For this review, take the finished solid that the model builds, in its own axes (mm). Round coordinates to 2 decimals unless told otherwise and drop trailing zeros. Write each loop counter-clockwise with the first axis right and the second up, starting at its lowest first coordinate (ties: lowest second). Pieces come first, ordered by that corner, then holes. Notation, with made-up numbers: M 50.25,-22.75 L 66.25,-22.75 A11 ccw 66.25,-14.75 Z; hole C -3.5,-0.75 d5. An arc over 180 degrees is marked long. Use one line per item in the form item = value. Start each with the question number.
Item 1: Add section D-D (z = -92). State the section outline as (x, y) points (3 decimals), and give its area (3 significant figures).
Item 2: Add section A-A (y = 1.75). Count the separate pieces of the cut face and the enclosed holes in it, and give its area (3 significant figures).
Item 3: Add section C-C (x = -102). State the section outline as (y, z) points, and give its area (3 significant figures).
Item 4: Add section B-B (z = 27.5). State the section outline as (x, y) points.
Item 5: For P1, Ø3, axis at x = -133.35, z = -133.35, coming from the +Y side, flat-tipped, find the tip position at first contact; note if it passes through.
Item 6: For line 1 (X direction, y = 4.25, z = 5); line 2 (X direction, y = 2.55, z = -133.35); line 3 (X direction, y = 5.5, z = 98.5) (3 decimals), list the stretches that pass through material, from the lowest coordinate up. Write a range as [from, to].
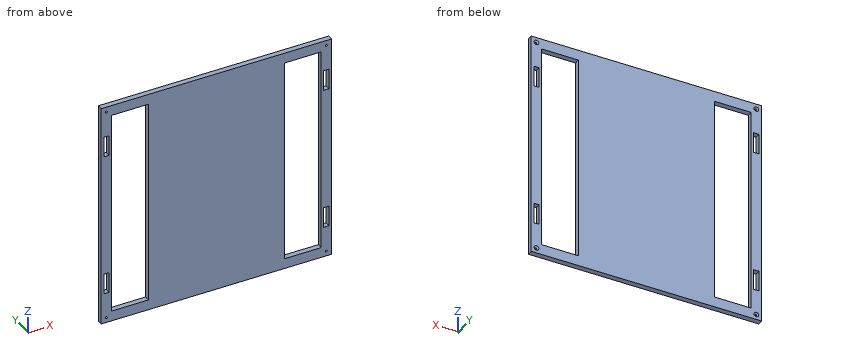
from build123d import *

# Parameters (mm, degrees)
SKETCH1_W                       = 279.4
SKETCH1_H                       = 279.4
BOSS_EXTRUDE1_DEPTH             = 6.35
SKETCH2_W                       = 44.45
SKETCH2_H                       = 254
SKETCH2_W_2                     = 6.35
SKETCH2_H_2                     = 25.4
CUT_EXTRUDE1_DEPTH              = 7.35
F_4_40_TAPPED_HOLE1_D           = 2.2606
F_4_40_TAPPED_HOLE1_CSINK_D     = 5.715
F_4_40_TAPPED_HOLE1_CSINK_ANGLE = 100


with BuildPart() as part:
    # Sketch1 → Boss-Extrude1 (new body)
    with BuildSketch(Plane(origin=(0, 0, 0), x_dir=(1, 0, 0), z_dir=(0, 1, 0))):
        Rectangle(SKETCH1_W, SKETCH1_H)
    extrude(amount=BOSS_EXTRUDE1_DEPTH)

    # Sketch2 → Cut-Extrude1 (cut, through all)
    with BuildSketch(Plane(origin=(0, 6.35, 0), x_dir=(1, 0, 0), z_dir=(0, 1, 0))):
        with Locations((-104.775, 0)):
            Rectangle(SKETCH2_W, SKETCH2_H)
        with Locations((104.775, 0)):
            Rectangle(SKETCH2_W, SKETCH2_H)
        with Locations((133.35, 88.9)):
            Rectangle(SKETCH2_W_2, SKETCH2_H_2)
        with Locations((-133.35, 88.9)):
            Rectangle(SKETCH2_W_2, SKETCH2_H_2)
        with Locations((133.35, -88.9)):
            Rectangle(SKETCH2_W_2, SKETCH2_H_2)
        with Locations((-133.35, -88.9)):
            Rectangle(SKETCH2_W_2, SKETCH2_H_2)
    extrude(amount=-CUT_EXTRUDE1_DEPTH, mode=Mode.SUBTRACT)

    # #4-40 Tapped Hole1 (through all)
    with Locations(Plane(origin=(0, 6.35, 0), x_dir=(1, 0, 0), z_dir=(0, 1, 0))):
        with Locations((-133.35, 133.35), (-133.35, -133.35), (133.35, -133.35), (133.35, 133.35)):
            CounterSinkHole(F_4_40_TAPPED_HOLE1_D / 2, F_4_40_TAPPED_HOLE1_CSINK_D / 2, counter_sink_angle=F_4_40_TAPPED_HOLE1_CSINK_ANGLE)


solid = part.part
Calculated:
q1.outline = M -139.7,0 L -136.525,0 L -136.525,6.35 L -139.7,6.35 Z; M -130.175,0 L -127,0 L -127,6.35 L -130.175,6.35 Z; M -82.55,0 L 82.55,0 L 82.55,6.35 L -82.55,6.35 Z; M 127,0 L 130.175,0 L 130.175,6.35 L 127,6.35 Z; M 136.525,0 L 139.7,0 L 139.7,6.35 L 136.525,6.35 Z
q1.area = 1,130 mm^2
q2.separate_pieces = 1
q2.enclosed_holes = 10
q2.area = 54,800 mm^2
q3.outline = M 0,-139.7 L 6.35,-139.7 L 6.35,-127 L 0,-127 Z; M 0,127 L 6.35,127 L 6.35,139.7 L 0,139.7 Z
q3.area = 161 mm^2
q4.outline = M -139.7,0 L -127,0 L -127,6.35 L -139.7,6.35 Z; M -82.55,0 L 82.55,0 L 82.55,6.35 L -82.55,6.35 Z; M 127,0 L 139.7,0 L 139.7,6.35 L 127,6.35 Z
q5.P1 = 5.21
q6.line_1 = [-139.7, -127], [-82.55, 82.55], [127, 139.7]
q6.line_2 = [-139.7, -134.48], [-132.22, 132.22], [134.48, 139.7]
q6.line_3 = [-139.7, -136.525], [-130.175, -127], [-82.55, 82.55], [127, 130.175], [136.525, 139.7]
